Read the model definition and answer for the solid it produces. Units are mm, in the model's axes. Give positions to 0.01 mm unless a question says otherwise; leave off trailing zeros. Order: outer loops, then holes, each group sorted by start corner. A loop starts at its lowest first (then second) coordinate and runs counter-clockwise, first axis right, second up. Notation, with made-up numbers: (-10, 23.5) - (32, 23.5) arc R14 cw to (32, 44.5) - close; hole circle Ø7 at (9, 21). An arc over 180 degrees is marked (long way). Write item = value, one per line.
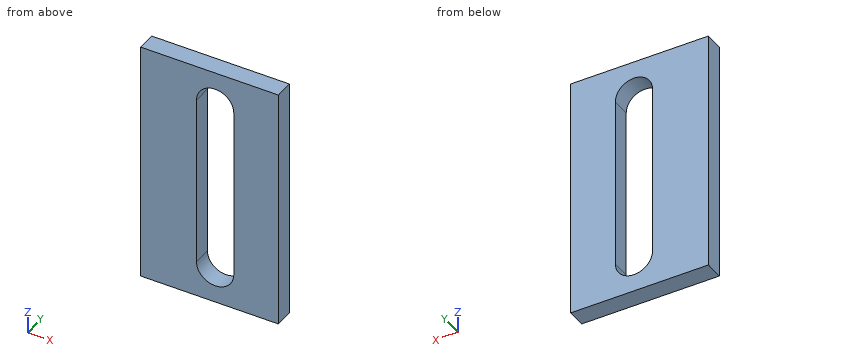
```python
from build123d import *

# Parameters (mm, degrees)
SKETCH1_W               = 13.8
SKETCH1_H               = 8.8
BOSS_EXTRUDE1_DEPTH     = 3
SKETCH2_W               = 2
SKETCH2_H               = 35
BOSS_EXTRUDE2_DEPTH     = 3
SKETCH3_W               = 1.2
SKETCH3_H               = 6
BOSS_EXTRUDE3_DEPTH     = 7
FILLET3_R               = 10
SKETCH5_W               = 15
SKETCH5_H               = 13.8
BOSS_EXTRUDE4_DEPTH     = 4
SKETCH6_R               = 1.5
CUT_EXTRUDE4_DEPTH      = 38.968539608
BOSS_EXTRUDE5_DEPTH     = 2
CHAMFER2_SIZE           = 3
BOSS_EXTRUDE7_DEPTH     = 1.2
SKETCH12_W              = 15
SKETCH12_H              = 4
BOSS_EXTRUDE8_DEPTH     = 3
SKETCH13_W              = 15
SKETCH13_H              = 4
BOSS_EXTRUDE9_DEPTH     = 3
CUT_EXTRUDE7_DEPTH      = 43.28486727
CUT_EXTRUDE7_DEPTH_BACK = 43.28486727
CUT_EXTRUDE8_DEPTH      = 43.28486727
CUT_EXTRUDE8_DEPTH_BACK = 43.28486727
SKETCH15_W              = 0.807911756
SKETCH15_H              = 0.64
CUT_EXTRUDE9_DEPTH      = 41.244591358
CUT_EXTRUDE9_DEPTH_BACK = 41.244591358
SKETCH16_W              = 0.64
SKETCH16_H              = 0.6
CHAMFER3_SIZE           = 1
SKETCH18_W              = 20.701942652
SKETCH18_H              = 41.728044518
CUT_EXTRUDE10_DEPTH     = 36
SKETCH19_W              = 11.097134513
SKETCH19_H              = 20.928514419
CUT_EXTRUDE11_DEPTH     = 2.5


# Some blends are built 0.0001 mm under size
with BuildPart() as part:
    # Sketch1 → Boss-Extrude1 (new body)
    with BuildSketch(Plane(origin=(0, 0, 0), x_dir=(0, 0, -1), z_dir=(1, 0, 0))):
        Rectangle(SKETCH1_W, SKETCH1_H)
    extrude(amount=BOSS_EXTRUDE1_DEPTH)

    # Sketch2 → Boss-Extrude2 (add)
    with BuildSketch(Plane(origin=(3, 0, 0), x_dir=(0, 0, -1), z_dir=(1, 0, 0))):
        with Locations((0, -13.1)):
            Rectangle(SKETCH2_W, SKETCH2_H)
    extrude(amount=BOSS_EXTRUDE2_DEPTH)

    # Sketch3 → Boss-Extrude3 (add)
    with BuildSketch(Plane(origin=(6, 0, 0), x_dir=(0, 0, -1), z_dir=(1, 0, 0))):
        with Locations((0, -27.6)):
            Rectangle(SKETCH3_W, SKETCH3_H)
    extrude(amount=BOSS_EXTRUDE3_DEPTH)

    # Fillet3
    # the kernel refuses this fillet: 10 mm, written as the material it adds along each edge
    with BuildSketch(Plane(origin=(3, -4.4, 1), x_dir=(-1, 0, 0), z_dir=(0, 0, -1))) as fillet3_piece_1:
        with BuildLine():
            CenterArc((10, -7.141428429), FILLET3_R, 134.427004001, 45.572995999)
            Line((0, -7.141428429), (0, 0))
            Line((0, 0), (3, 0))
        make_face()
    extrude(amount=2)

    # Sketch5 → Boss-Extrude4 (add)
    with BuildSketch(Plane(origin=(0, 4.4, 0), x_dir=(1, 0, 0), z_dir=(0, 1, 0))):
        with Locations((-4.5, 0)):
            Rectangle(SKETCH5_W, SKETCH5_H)
    extrude(amount=BOSS_EXTRUDE4_DEPTH)

    # Sketch6 → Cut-Extrude4 (cut, through all)
    with BuildSketch(Plane.XZ.offset(-4.4)):
        with Locations(Location((-6, 3, 0), (0, 0, 270))):
            Circle(SKETCH6_R)
        with Locations(Location((-6, -3, 0), (0, 0, 270))):
            Circle(SKETCH6_R)
    extrude(amount=-CUT_EXTRUDE4_DEPTH, mode=Mode.SUBTRACT)

    # Sketch8 → Boss-Extrude5 (add)
    with BuildSketch(Plane(origin=(0, 0, -1), x_dir=(-1, 0, 0), z_dir=(0, 0, -1))):
        Polygon((-3, -18.758153574), (0, -4.4), (-3, -4.4), align=None)
    extrude(amount=-BOSS_EXTRUDE5_DEPTH)

    # Chamfer2
    chamfer2_edges = [part.edges().sort_by_distance(p)[0] for p in [
        (3, 4.4, 0),
    ]]
    chamfer(chamfer2_edges, length=CHAMFER2_SIZE - 0.0001)  # a hair under: the kernel refuses the full size

    # Sketch11 → Boss-Extrude7 (add)
    with BuildSketch(Plane(origin=(0, 0, -0.6), x_dir=(-1, 0, 0), z_dir=(0, 0, -1))):
        Polygon((-6, -24.6), (-13, -24.6), (-6, 1.742521041), align=None)
    extrude(amount=-BOSS_EXTRUDE7_DEPTH)

    # Sketch12 → Boss-Extrude8 (add)
    with BuildSketch(Plane(origin=(0, 0, -6.9), x_dir=(-1, 0, 0), z_dir=(0, 0, -1))):
        with Locations((4.5, 6.4)):
            Rectangle(SKETCH12_W, SKETCH12_H)
    extrude(amount=BOSS_EXTRUDE8_DEPTH)

    # Sketch13 → Boss-Extrude9 (add)
    with BuildSketch(Plane.XY.offset(6.9)):
        with Locations((-4.5, 6.4)):
            Rectangle(SKETCH13_W, SKETCH13_H)
    extrude(amount=BOSS_EXTRUDE9_DEPTH)

    # Sketch14 → Cut-Extrude7 (cut, two sides: drawn at the far end of the back side and taken through both)
    with BuildSketch(Plane(origin=(0, 8.4, 0), x_dir=(1, 0, 0), z_dir=(0, 1, 0)).offset(-CUT_EXTRUDE7_DEPTH_BACK)):
        with BuildLine():
            Line((-7.5, 7), (-7.5, -7))
            ThreePointArc((-7.5, -7), (-6, -8.5), (-4.5, -7))
            Line((-4.5, -7), (-4.5, 7))
            ThreePointArc((-4.5, 7), (-6, 8.5), (-7.5, 7))
        make_face()
    extrude(amount=CUT_EXTRUDE7_DEPTH + CUT_EXTRUDE7_DEPTH_BACK, mode=Mode.SUBTRACT)

    # Sketch15 → Cut-Extrude8 (cut, two sides: drawn at the far end of the back side and taken through both)
    with BuildSketch(Plane.XZ.offset(30.6).offset(-CUT_EXTRUDE8_DEPTH_BACK)):
        with Locations((12.596044122, 0)):
            Rectangle(SKETCH15_W, SKETCH15_H)
    extrude(amount=CUT_EXTRUDE8_DEPTH + CUT_EXTRUDE8_DEPTH_BACK, mode=Mode.SUBTRACT)

    # Sketch16 → Cut-Extrude9 (cut, two sides: drawn at the far end of the back side and taken through both)
    with BuildSketch(Plane(origin=(12.192088244, 0, 0), x_dir=(0, 0, -1), z_dir=(1, 0, 0)).offset(-CUT_EXTRUDE9_DEPTH_BACK)):
        with Locations((0, -30.3)):
            Rectangle(SKETCH16_W, SKETCH16_H)
    extrude(amount=CUT_EXTRUDE9_DEPTH + CUT_EXTRUDE9_DEPTH_BACK, mode=Mode.SUBTRACT)

    # Chamfer3
    chamfer3_edges = [part.edges().sort_by_distance(p)[0] for p in [
        (12.192088244, -30, 0),
    ]]
    chamfer(chamfer3_edges, length=CHAMFER3_SIZE)

    # Sketch18 → Cut-Extrude10 (cut)
    with BuildSketch(Plane.XY.offset(9.9)):
        with Locations((9.448105839, -12.464022259)):
            Rectangle(SKETCH18_W, SKETCH18_H)
    extrude(amount=-CUT_EXTRUDE10_DEPTH, mode=Mode.SUBTRACT)

    # Sketch19 → Cut-Extrude11 (cut)
    with BuildSketch(Plane.XZ.offset(-4.4)):
        with Locations((-6.451432743, 0.56425721)):
            Rectangle(SKETCH19_W, SKETCH19_H)
    extrude(amount=-CUT_EXTRUDE11_DEPTH, mode=Mode.SUBTRACT)


solid = part.part
```
1. A flat-ended cylindrical pin translates along its axis: pin 1 (3 mm diameter, centred on x = -7, z = -3, fed in from +Y). Find the tip coordinate at first contact, or state that the pin passes through.
Recorded:
pin_1 = 8.4
2. Straight lines are drawn through the part: L1, parallel to X at y = 7.7, z = 4.5; L2, parallel to Z at x = -7.25, y = 7.4; L3, parallel to Z at x = -7, y = 8.05. For each, find the intervals that lie inside material, in ascending order. Write a range as [from, to].
Recorded:
L1 = [-12, -7.5], [-4.5, -0.9]
L2 = [-9.9, -7.83], [7.83, 9.9]
L3 = [-9.9, -8.12], [8.12, 9.9]
3. Section B-B (z = -3.5) is taken. Determine the outline of the cut face in (x, y).
Recorded:
outline = (-12, 6.9) - (-7.5, 6.9) - (-7.5, 8.4) - (-12, 8.4) - close; (-4.5, 6.9) - (-0.9, 6.9) - (-0.9, 8.4) - (-4.5, 8.4) - close
4. Section C-C (y = 7.95) is taken. Determine the outline of the cut face in (x, z).
Recorded:
outline = (-12, -9.9) - (-0.9, -9.9) - (-0.9, 9.9) - (-12, 9.9) - close; hole (-7.5, -7) arc R1.5 ccw to (-4.5, -7) - (-4.5, 7) arc R1.5 ccw to (-7.5, 7) - close
5. Section A-A (x = -6) is taken. Determine the outline of the cut face in (y, z), and give its area (3 significant figures).
Recorded:
outline = (6.9, -9.9) - (8.4, -9.9) - (8.4, -8.5) - (6.9, -8.5) - close; (6.9, 8.5) - (8.4, 8.5) - (8.4, 9.9) - (6.9, 9.9) - close
area = 4.20 mm^2
